Could you check a few things on this model? Use its own coordinates, in mm. Round coordinates to 2 decimals unless told otherwise and drop trailing zeros. Write each loop counter-clockwise with the first axis right and the second up, starting at its lowest first coordinate (ties: lowest second). Pieces come first, ordered by that corner, then holes. Notation, with made-up numbers: (73, -39) -> (116, -39) arc R11 ccw to (116, -29) -> close; hole circle Ø7 at (1.5, -2). An arc over 180 degrees is marked (long way). Answer as CSV lines item,"result". Start each with the question number.
Q1. If I drill on line 1 (Y direction, x = 1.25, z = 1.7); line 2 (X direction, y = -1.75, z = 1.1); line 3 (Y direction, x = 21.25, z = 1.6), over which ranges is the centre line in solid material (lowest first)? Write a range as [from, to].
Q2. Will these pins go through, and if not, where does the flat tip stop? pin 1 Ø1 at (x, z) = (37.5, 1.5) entering from +Y; pin 2 Ø1.4 at (y, z) = (1.5, 1.5) entering from -X; pin 3 Ø0.6 at (y, z) = (-0.5, 2) entering from -X.
Q3. Imagine slicing it at A-A on x = 15. Please give me the cut outline in (y, z), and give its area (3 significant figures).
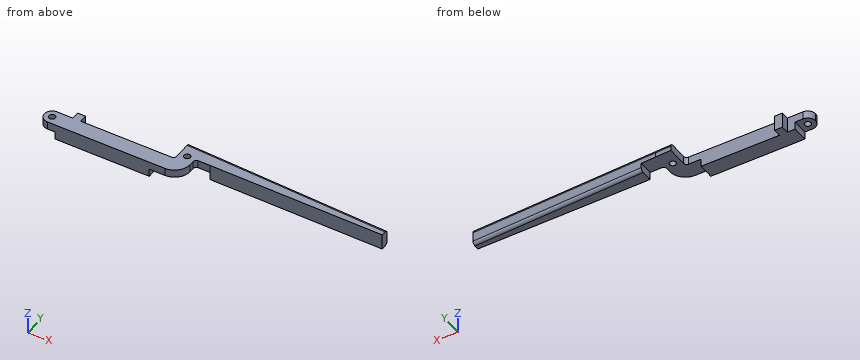
from build123d import *

# Parameters (mm, degrees)
BOSS_EXTRUDE1_DEPTH = 2.5
SKETCH2_W           = 2.5
SKETCH2_H           = 6.25
SKETCH2_H_2         = 2.5
CUT_EXTRUDE1_DEPTH  = 1.25
SKETCH3_R           = 0.5
CUT_EXTRUDE2_DEPTH  = 2.25
SKETCH4_W           = 2.5
SKETCH4_H           = 2.5
SKETCH4_R           = 0.5
SKETCH4_H_2         = 6.134615385
BOSS_EXTRUDE2_DEPTH = 1.25
BOSS_EXTRUDE3_DEPTH = 1.25
SKETCH6_W           = 2.5
SKETCH6_H           = 6.25
SKETCH6_H_2         = 2.5
CUT_EXTRUDE3_DEPTH  = 1.25
CUT_EXTRUDE4_DEPTH  = 1.25
CUT_EXTRUDE5_DEPTH  = 1.25
CUT_EXTRUDE6_DEPTH  = 1.25
CUT_EXTRUDE7_DEPTH  = 1.25
CUT_EXTRUDE8_DEPTH  = 1.25
BOSS_EXTRUDE4_DEPTH = 1.25
CUT_EXTRUDE9_DEPTH  = 1.25
FILLET2_R           = 0.5
FILLET3_R           = 0.5
FILLET4_R           = 0.5
CUT_EXTRUDE10_DEPTH = 1.25
SKETCH16_W          = 2.5
SKETCH16_H          = 2.5
BOSS_EXTRUDE5_DEPTH = 1.25
SKETCH17_W          = 27.617920392
SKETCH17_H          = 2.5
BOSS_EXTRUDE6_DEPTH = 0.25
CUT_EXTRUDE11_DEPTH = 3.5
SKETCH19_W          = 1.25
SKETCH19_H          = 1.25
CUT_EXTRUDE12_DEPTH = 3.5


with BuildPart() as part:
    # Sketch1 → Boss-Extrude1 (new body)
    with BuildSketch(Plane.XY):
        Polygon((0, -1.25), (0, -3.75), (20, -3.75), (22.5, -3.75), (22.5, 0), (52.5, 0), (52.5, 1), (20, 2.5), (20, 0), (20, -1.25), align=None)
    extrude(amount=BOSS_EXTRUDE1_DEPTH)

    # Sketch2 → Cut-Extrude1 (cut)
    with BuildSketch(Plane.XY.offset(2.5)):
        with Locations((21.25, -0.625)):
            Rectangle(SKETCH2_W, SKETCH2_H)
        with Locations((1.25, -2.5)):
            Rectangle(SKETCH2_W, SKETCH2_H_2)
    extrude(amount=-CUT_EXTRUDE1_DEPTH, mode=Mode.SUBTRACT)

    # Sketch3 → Cut-Extrude2 (cut, through all)
    with BuildSketch(Plane.XY.offset(1.25)):
        with Locations((1.25, -2.5)):
            Circle(SKETCH3_R)
        with Locations((21.25, 0)):
            Circle(SKETCH3_R)
    extrude(amount=-CUT_EXTRUDE2_DEPTH, mode=Mode.SUBTRACT)

    # Sketch4 → Boss-Extrude2 (add)
    with BuildSketch(Plane.XY.offset(1.25)):
        with Locations((1.25, -2.5)):
            Rectangle(SKETCH4_W, SKETCH4_H)
        with Locations((1.25, -2.5)):
            Circle(SKETCH4_R, mode=Mode.SUBTRACT)
        with Locations((21.25, -0.682692308)):
            Rectangle(SKETCH4_W, SKETCH4_H_2)
        with Locations((21.25, 0)):
            Circle(SKETCH4_R, mode=Mode.SUBTRACT)
    extrude(amount=BOSS_EXTRUDE2_DEPTH)

    # Sketch5 → Boss-Extrude3 (add)
    with BuildSketch(Plane.XY.offset(1.25)):
        Polygon((20, 2.384615385), (20, 2.5), (22.5, 2.384615385), align=None)
    extrude(amount=BOSS_EXTRUDE3_DEPTH)

    # Sketch6 → Cut-Extrude3 (cut)
    with BuildSketch(Plane(origin=(0, 0, 0), x_dir=(-1, 0, 0), z_dir=(0, 0, -1))):
        with Locations((-21.25, -0.625)):
            Rectangle(SKETCH6_W, SKETCH6_H)
        with Locations((-1.25, -2.5)):
            Rectangle(SKETCH6_W, SKETCH6_H_2)
    extrude(amount=-CUT_EXTRUDE3_DEPTH, mode=Mode.SUBTRACT)

    # Sketch7 → Cut-Extrude4 (cut)
    with BuildSketch(Plane(origin=(0, 0, 0), x_dir=(-1, 0, 0), z_dir=(0, 0, -1))):
        with BuildLine():
            Line((-2.5, -3.75), (-2.5, -1.25))
            ThreePointArc((-2.5, -1.25), (-3.75, -2.5), (-2.5, -3.75))
        make_face()
    extrude(amount=-CUT_EXTRUDE4_DEPTH, mode=Mode.SUBTRACT)

    # Sketch9 → Cut-Extrude5 (cut)
    with BuildSketch(Plane(origin=(0, 0, 1.25), x_dir=(-1, 0, 0), z_dir=(0, 0, -1))):
        with BuildLine():
            Line((0, -1.25), (-1.25, -1.25))
            ThreePointArc((-1.25, -1.25), (-0.366116524, -1.616116524), (0, -2.5))
            Line((0, -2.5), (0, -1.25))
        make_face()
        with BuildLine():
            Line((0, -3.75), (0, -2.5))
            ThreePointArc((0, -2.5), (-0.366116524, -3.383883476), (-1.25, -3.75))
            Line((-1.25, -3.75), (0, -3.75))
        make_face()
    extrude(amount=-CUT_EXTRUDE5_DEPTH, mode=Mode.SUBTRACT)

    # Sketch10 → Cut-Extrude6 (cut)
    with BuildSketch(Plane(origin=(0, 0, 0), x_dir=(-1, 0, 0), z_dir=(0, 0, -1))):
        with BuildLine():
            Line((-22.5, 2.384615385), (-24.882079608, 2.274673249))
            ThreePointArc((-24.882079608, 2.274673249), (-24.146848631, 0.660005249), (-22.5, 0))
            Line((-22.5, 0), (-22.5, 2.384615385))
        make_face()
        with BuildLine():
            Line((-20, -3.75), (-20, -1.25))
            Line((-20, -1.25), (-17.5, -1.25))
            ThreePointArc((-17.5, -1.25), (-18.232233047, -3.017766953), (-20, -3.75))
        make_face()
    extrude(amount=-CUT_EXTRUDE6_DEPTH, mode=Mode.SUBTRACT)

    # Sketch11 → Cut-Extrude7 (cut)
    with BuildSketch(Plane(origin=(0, 0, 1.25), x_dir=(-1, 0, 0), z_dir=(0, 0, -1))):
        with BuildLine():
            Line((-22.5, -1.25), (-22.5, -3.75))
            Line((-22.5, -3.75), (-20, -3.75))
            ThreePointArc((-20, -3.75), (-21.767766953, -3.017766953), (-22.5, -1.25))
        make_face()
    extrude(amount=-CUT_EXTRUDE7_DEPTH, mode=Mode.SUBTRACT)

    # Sketch12 → Cut-Extrude8 (cut)
    with BuildSketch(Plane(origin=(0, 0, 0), x_dir=(-1, 0, 0), z_dir=(0, 0, -1))):
        with BuildLine():
            Line((-24.882079608, 2.274673249), (-24.882079608, 0))
            Line((-24.882079608, 0), (-22.5, 0))
            ThreePointArc((-22.5, 0), (-24.146848631, 0.660005249), (-24.882079608, 2.274673249))
        make_face()
    extrude(amount=-CUT_EXTRUDE8_DEPTH, mode=Mode.SUBTRACT)

    # Sketch13 → Boss-Extrude4 (add)
    with BuildSketch(Plane(origin=(0, 0, 1.25), x_dir=(-1, 0, 0), z_dir=(0, 0, -1))):
        with BuildLine():
            Line((-2.5, -1.25), (-2, -1.25))
            ThreePointArc((-2, -1.25), (-2.5, -2.5), (-2, -3.75))
            Line((-2, -3.75), (-2.5, -3.75))
            ThreePointArc((-2.5, -3.75), (-3.75, -2.5), (-2.5, -1.25))
        make_face()
    extrude(amount=BOSS_EXTRUDE4_DEPTH)

    # Sketch14 → Cut-Extrude9 (cut)
    with BuildSketch(Plane(origin=(0, 0, 0), x_dir=(-1, 0, 0), z_dir=(0, 0, -1))):
        with BuildLine():
            Line((-17.5, -1.25), (-17.5, -3.75))
            Line((-17.5, -3.75), (-20, -3.75))
            ThreePointArc((-20, -3.75), (-18.232233047, -3.017766953), (-17.5, -1.25))
        make_face()
    extrude(amount=-CUT_EXTRUDE9_DEPTH, mode=Mode.SUBTRACT)

    # Fillet2
    fillet2_edges = [part.edges().sort_by_distance(p)[0] for p in [
        (38.691039804, 1.637336624, 0),
        (36.25, 1.75, 2.5),
    ]]
    fillet(fillet2_edges, radius=FILLET2_R)

    # Fillet3
    fillet3_edges = [part.edges().sort_by_distance(p)[0] for p in [
        (22.5, 0, 1.875),
    ]]
    fillet(fillet3_edges, radius=FILLET3_R)

    # Fillet4
    fillet4_edges = [part.edges().sort_by_distance(p)[0] for p in [
        (20, -1.25, 1.875),
    ]]
    fillet(fillet4_edges, radius=FILLET4_R)

    # Sketch15 → Cut-Extrude10 (cut)
    with BuildSketch(Plane(origin=(0, 0, 0), x_dir=(-1, 0, 0), z_dir=(0, 0, -1))):
        with BuildLine():
            Line((-2.5, -1.25), (-2.5, -2.500000004))
            ThreePointArc((-2.5, -2.500000004), (-2.370364003, -1.826854401), (-2, -1.25))
            Line((-2, -1.25), (-2.5, -1.25))
        make_face()
        with BuildLine():
            Line((-2.5, -3.75), (-2, -3.75))
            ThreePointArc((-2, -3.75), (-2.370364002, -3.173145603), (-2.5, -2.500000004))
            Line((-2.5, -2.500000004), (-2.5, -3.75))
        make_face()
    extrude(amount=-CUT_EXTRUDE10_DEPTH, mode=Mode.SUBTRACT)

    # Sketch16 → Boss-Extrude5 (add)
    with BuildSketch(Plane(origin=(0, -1.25, 0), x_dir=(1, 0, 0), z_dir=(0, 1, 0))):
        with Locations((3.75, -1.25)):
            Rectangle(SKETCH16_W, SKETCH16_H)
    extrude(amount=BOSS_EXTRUDE5_DEPTH)

    # Sketch17 → Boss-Extrude6 (add)
    with BuildSketch(Plane.XZ):
        with Locations((38.691039804, 1.25)):
            Rectangle(SKETCH17_W, SKETCH17_H)
    extrude(amount=BOSS_EXTRUDE6_DEPTH)

    # Sketch18 → Cut-Extrude11 (cut, through all)
    with BuildSketch(Plane(origin=(0, 0, 0), x_dir=(-1, 0, 0), z_dir=(0, 0, -1))):
        Polygon((-24.882079608, 0), (-52.5, -0.25), (-24.882079608, -0.25), align=None)
    extrude(amount=-CUT_EXTRUDE11_DEPTH, mode=Mode.SUBTRACT)

    # Sketch19 → Cut-Extrude12 (cut, through all)
    with BuildSketch(Plane(origin=(0, 0, 0), x_dir=(-1, 0, 0), z_dir=(0, 0, -1))):
        with Locations((-3.125, -0.625)):
            Rectangle(SKETCH19_W, SKETCH19_H)
    extrude(amount=-CUT_EXTRUDE12_DEPTH, mode=Mode.SUBTRACT)


solid = part.part
Checks:
1,line 1,"[-3.75, -3], [-2, -1.25]"
1,line 2,"[2.5, 17.5]"
1,line 3,"[-3.42, -0.5], [0.5, 2.44]"
2,pin 1,"y = 1.72"
2,pin 2,"x = 20"
2,pin 3,"x = 3.75"
3,outline,"(-3.75, 0) -> (-1.25, 0) -> (-1.25, 2.5) -> (-3.75, 2.5) -> close"
3,area,"6.25 mm^2"
